```python
from build123d import *

# Parameters (mm, degrees)
SKETCH_1_R          = 30
SKETCH_1_R_2        = 20
SKETCH_1_R_3        = 1.1
EXTRUDE_1_DEPTH     = 5
CUT_EXTRUDE_START   = -10
CUT_EXTRUDE_1_DEPTH = 10
FILLET_1_R          = 2


with BuildPart() as part:
    # 草图1 → 凸台-拉伸1 (new body)
    with BuildSketch(Plane(origin=(0, 0, 0), x_dir=(1, 0, 0), z_dir=(0, 1, 0))):
        with Locations(Location((0, 0, 0), (0, 0, 270))):
            Circle(SKETCH_1_R)
        with Locations(Location((0, 0, 0), (0, 0, 270))):
            Circle(SKETCH_1_R_2, mode=Mode.SUBTRACT)
        with Locations(Location((0, 24.5, 0), (0, 0, 270))):
            Circle(SKETCH_1_R_3, mode=Mode.SUBTRACT)
        with Locations(Location((21.217622393, -12.25, 0), (0, 0, 270))):
            Circle(SKETCH_1_R_3, mode=Mode.SUBTRACT)
        with Locations(Location((-21.217622393, -12.25, 0), (0, 0, 270))):
            Circle(SKETCH_1_R_3, mode=Mode.SUBTRACT)
    extrude(amount=EXTRUDE_1_DEPTH)

    # 草图2 → 切除-拉伸1 (cut)
    with BuildSketch(Plane(origin=(0, 5, 0), x_dir=(1, 0, 0), z_dir=(0, 1, 0)).offset(CUT_EXTRUDE_START)):
        with BuildLine():
            Line((19.339127693, -22.934649334), (14.401131779, -13.878306939))
            ThreePointArc((14.401131779, -13.878306939), (0.907800118, -19.979386851), (-13.08321747, -15.1271088))
            Line((-13.08321747, -15.1271088), (-17.179578816, -24.593943801))
            ThreePointArc((-17.179578816, -24.593943801), (1.361700176, -29.969080277), (19.339127693, -22.934649334))
        make_face()
    extrude(amount=CUT_EXTRUDE_1_DEPTH, mode=Mode.SUBTRACT)

    # 圆角1
    fillet_1_edges = [part.edges().sort_by_distance(p)[0] for p in [
        (14.401131779, 2.5, 13.878306939),
        (-13.08321747, 2.5, 15.1271088),
        (19.339127693, 2.5, 22.934649334),
        (-17.179578816, 2.5, 24.593943801),
    ]]
    fillet(fillet_1_edges, radius=FILLET_1_R)


solid = part.part
```
Part model, mm, in its own coordinate system. A direction names the side the tool comes from. Round coordinates to 2 decimals unless told otherwise and drop trailing zeros. Loops run counter-clockwise (first coordinate to the right, second up) from the corner with the lowest first, then second, coordinate; pieces in that order, holes last.
Item 1: Cut at B-B, the plane z = 0. Give the cut face in (x, y), then the cut area to 3 significant figures.
Item 2: Drill centre lines: line 1 (X direction, y = 0.3, z = 0.5); line 2 (X direction, y = 3.4, z = 12.25); line 3 (X direction, y = 0.7, z = -5). Where is each one in solid material? Low to high.
Item 3: Cut at D-D, the plane x = 11. Give the cut face in (y, z), then the cut area to 3 significant figures.
Item 4: Drop flat-ended pins along their axis: P1, Ø1.8, axis at x = 0, z = -24.5, coming from the -Y side; P2, Ø3, axis at x = -0.5, y = 1.5, coming from the +Z side; P3, Ø3, axis at x = 8, y = 2, coming from the +Z side. Give the stop position or say it passes through.
Item 5: 3-axis set-ups, long thin cutter, end or side, ignore diameter. For faces 4 (the face through (14.843, 2.535, 13.98)), 5 (the face through (0, 0, -21)), 6 (the face through (-14.886, 2.465, 19.294)): which of +Z, -Z, +X, -X, +Y, -Y reach the whole face in a straight line?
Item 6: Cut at C-C, the plane y = 2.6. Give the cut face in (x, z), then the cut area to 3 significant figures.
Item 7: Mould opens along X. For faces 1 (the face through (-17.56, 2.54, 23.4)), 2 (the face through (0, 5, -21)), 3 (the face through (0, 2, -20)) say: +X half, -X half, draft (parallel to the pull), parting line (faces both ways), or undercut.
Item 8: Cut at A-A, the plane x = 0. Give the cut face in (y, z), then the cut area to 3 significant figures.
A:
1. outline: (-30, 0) - (-20, 0) - (-20, 5) - (-30, 5) - close; (20, 0) - (30, 0) - (30, 5) - (20, 5) - close
1. area: 100 mm2
2. line 1: x = -30 to -19.99, 19.99 to 30
2. line 2: x = -27.38 to -22.32, -20.12 to -15.81, 15.81 to 20.12, 22.32 to 27.38
2. line 3: x = -29.58 to -19.36, 19.36 to 29.58
3. outline: (0, -27.91) - (5, -27.91) - (5, -16.7) - (0, -16.7) - close
3. area: 56.0 mm2
4. P1: passes through
4. P2: stops at z = -19.9
4. P3: stops at z = -17.6
5. face 4: +Y, -Y
5. face 5: +Z, -Z, +X, -X, -Y
5. face 6: +Z, +Y, -Y
6. outline: (-19.28, 22.98) arc R30 ccw (long way) to (21.29, 21.14) arc R2 ccw to (18.11, 20.69) - (15.08, 15.12) arc R2 ccw to (15.3, 12.88) arc R20 cw (long way) to (-14.07, 14.21) arc R2 ccw to (-13.65, 16.43) - (-16.16, 22.24) arc R2 ccw to start; hole circle Ø2.2 at (-21.22, 12.25); hole circle Ø2.2 at (0, -24.5); hole circle Ø2.2 at (21.22, 12.25)
6. area: 1,210 mm2
7. face 1: parting line
7. face 2: draft
7. face 3: undercut
8. outline: (0, -30) - (5, -30) - (5, -25.6) - (0, -25.6) - close; (0, -23.4) - (5, -23.4) - (5, -20) - (0, -20) - close
8. area: 39.0 mm2
